Answer from the drawing. Dimensions are ordinates in mm from the lowest x, y and z of the part. Give positions to 0.01 mm unless a question says otherwise; leave off trailing zeros. Write each loop counter-clockwise with the first axis right and the second up, starting at its lowest first coordinate (ties: lowest second). Pieces come first, ordered by that corner, then holes. Notation, with made-up numbers: (85.25, 4.5) -> (90.25, 4.5) arc R32 cw to (90.25, 41.5) -> close; hole circle Ø5 at (-25, 39.5). An arc over 180 degrees is marked (long way). Use a Markdown table: item, result. Add a question column.
Q1. Consider line 1 (X direction, y = 58.5, z = 9.75); line 2 (X direction, y = 37, z = 11.25); line 3 (Y direction, x = 314.5, z = 1.25). Determine where each line is inside the solid, lowest interval first.
Q2. Section D-D, the plane y = 5 is taken. Give the vertices of the cut face in (x, z), plus the area to 3 significant figures.
Q3. Section C-C, the plane x = 312 is taken. Give the vertices of the cut face in (y, z).
Q4. Each of these flat-tipped pins is pushed along its axis until it touches: pin 1 Ø4 at (x, z) = (97.5, 5.5) entering from +Y; pin 2 Ø6 at (y, z) = (57.5, 7.5) entering from +X; pin 3 Ø4 at (y, z) = (42.5, 10.5) entering from -X; pin 4 Ø1.5 at (x, z) = (78, 8) entering from -Y. Where does it stop, or does it pass through?
Q5. Section A-A, the plane y = 54 is taken. Give the vertices of the cut face in (x, z), plus the area to 3 significant figures.
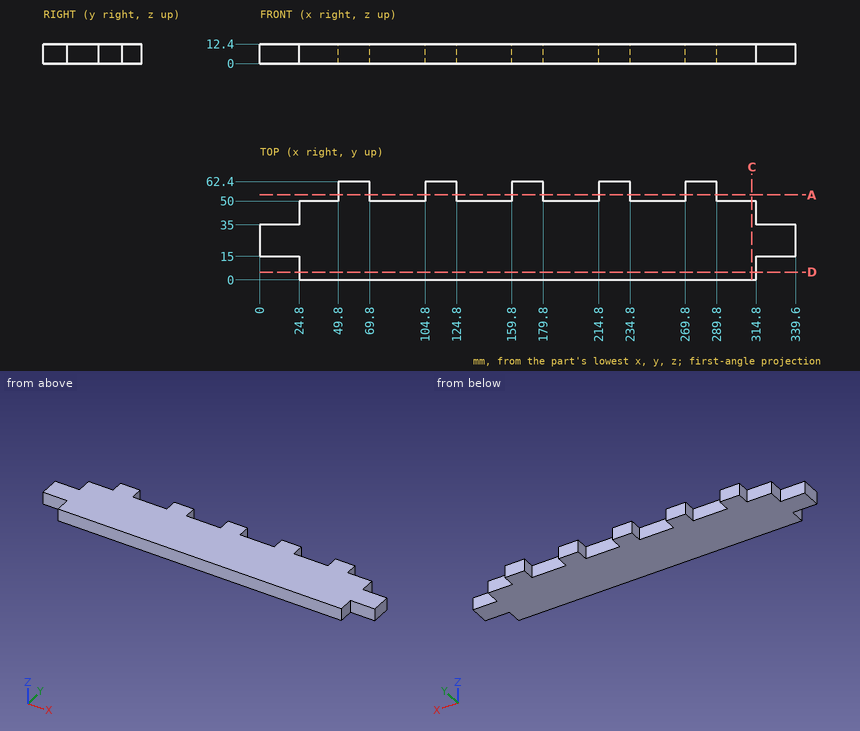
Result set:
| question | item | result |
|---|---|---|
| 1 | line 1 | x = 49.8 to 69.8, 104.8 to 124.8, 159.8 to 179.8, 214.8 to 234.8, 269.8 to 289.8 |
| 1 | line 2 | x = 24.8 to 314.8 |
| 1 | line 3 | y = 0 to 50 |
| 2 | outline | (24.8, 0) -> (314.8, 0) -> (314.8, 12.4) -> (24.8, 12.4) -> close |
| 2 | area | 3,600 mm2 |
| 3 | outline | (0, 0) -> (50, 0) -> (50, 12.4) -> (0, 12.4) -> close |
| 4 | pin 1 | stops at y = 50 |
| 4 | pin 2 | stops at x = 289.8 |
| 4 | pin 3 | stops at x = 24.8 |
| 4 | pin 4 | stops at y = 0 |
| 5 | outline | (49.8, 0) -> (69.8, 0) -> (69.8, 12.4) -> (49.8, 12.4) -> close; (104.8, 0) -> (124.8, 0) -> (124.8, 12.4) -> (104.8, 12.4) -> close; (159.8, 0) -> (179.8, 0) -> (179.8, 12.4) -> (159.8, 12.4) -> close; (214.8, 0) -> (234.8, 0) -> (234.8, 12.4) -> (214.8, 12.4) -> close; (269.8, 0) -> (289.8, 0) -> (289.8, 12.4) -> (269.8, 12.4) -> close |
| 5 | area | 1,240 mm2 |
